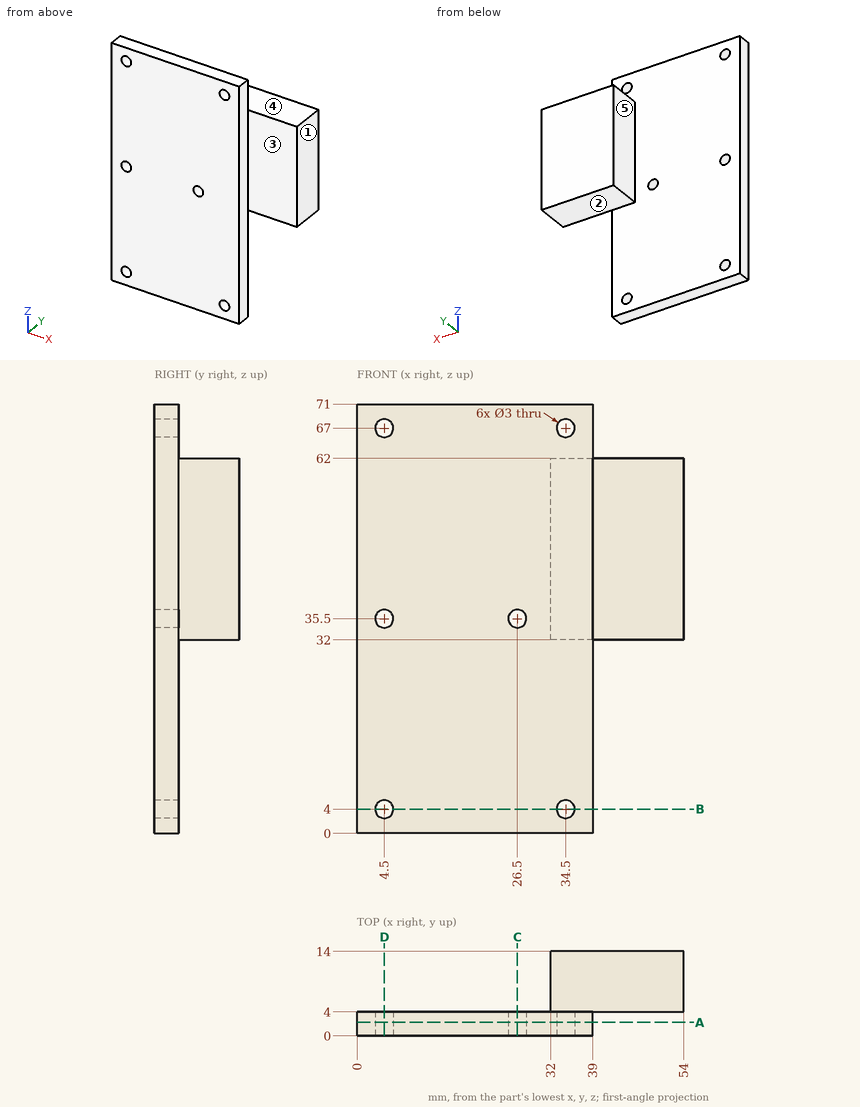
Geometry check sheet. Reference: drawing and pictorial views, mm from the part's lowest x, y, z. A direction names the side the tool comes from. Coordinates: 2 decimals unless noted, no trailing zeros. Order: outer loops, then holes, each group sorted by start corner. A loop starts at its lowest first (then second) coordinate and runs counter-clockwise, first axis right, second up. Notation, with made-up numbers: M 31,26.25 L 50,26.25 A24 cw 50,37.25 Z; hole C 20,9.5 d7. An arc over 180 degrees is marked long. Return JSON: item names as keys, results as strings.
1) Cross-section at C-C, the plane x = 26.5. Record the boundary of the cut face in (y, z).
Answer list:
{"outline": "M 0,0 L 4,0 L 4,34 L 0,34 Z; M 0,37 L 4,37 L 4,71 L 0,71 Z"}
2) Cross-section at A-A, the plane y = 2.25. Record the boundary of the cut face in (x, z), and give its area (3 significant figures).
Answer list:
{"outline": "M 0,0 L 39,0 L 39,71 L 0,71 Z; hole C 4.5,4 d3; hole C 4.5,35.5 d3; hole C 4.5,67 d3; hole C 26.5,35.5 d3; hole C 34.5,4 d3; hole C 34.5,67 d3", "area": "2,730 mm2"}
3) Access from +Z, -Z, +X, -X, +Y, -Y to the whole of each face (thin tool, end or side, straight path). Record for the marked faces 1, 2, 3, 4 and 5.
Answer list:
{"face 1": "+Z, -Z, +X, +Y, -Y", "face 2": "-Z, +X, -X, +Y", "face 3": "+Z, -Z, +X, -Y", "face 4": "+Z, +X, -X, +Y", "face 5": "+Z, -Z, -X, +Y"}
4) Cross-section at D-D, the plane x = 4.5. Record the boundary of the cut face in (y, z), and give its area (3 significant figures).
Answer list:
{"outline": "M 0,0 L 4,0 L 4,2.5 L 0,2.5 Z; M 0,5.5 L 4,5.5 L 4,34 L 0,34 Z; M 0,37 L 4,37 L 4,65.5 L 0,65.5 Z; M 0,68.5 L 4,68.5 L 4,71 L 0,71 Z", "area": "248 mm2"}
5) Cross-section at B-B, the plane z = 4. Record the boundary of the cut face in (x, y).
Answer list:
{"outline": "M 0,0 L 3,0 L 3,4 L 0,4 Z; M 6,0 L 33,0 L 33,4 L 6,4 Z; M 36,0 L 39,0 L 39,4 L 36,4 Z"}
6) Gauge pin test, flat ends, axial feed: pin 1 (8 mm diameter, centred on x = 46, y = 10.5, fed in from +Z); pin 2 (8 mm diameter, centred on x = 25, z = 21.5, fed in from +Y); pin 3 (5 mm diameter, centred on x = 37, y = 9.5, fed in from -Z); pin 4 (1.8 mm diameter, centred on x = 4.5, z = 67, fed in from -Y) (1 decimal). Record the tip position at first contact, or that the pin passes through.
Answer list:
{"pin 1": "z = 62", "pin 2": "y = 4", "pin 3": "z = 32", "pin 4": "through"}
7) Thickness scan on L1, parallel to X at y = 2.3, z = 4; L2, parallel to X at y = 2.15, z = 35.5; L3, parallel to Z at x = 4.5, y = 1.15. Record the ranges inside material, lowest first. Write a range as [from, to].
Answer list:
{"L1": "[0, 3], [6, 33], [36, 39]", "L2": "[0, 3], [6, 25], [28, 39]", "L3": "[0, 2.5], [5.5, 34], [37, 65.5], [68.5, 71]"}
